from build123d import *

# Parameters (mm, degrees)
SKETCH_W        = 100
SKETCH_H        = 64
SKETCH_R        = 10.1
SKETCH_R_2      = 1.8
SKETCH_R_3      = 3.2
SKETCH_R_4      = 4
PAD_DEPTH       = 15
SKETCH001_R     = 11.2
SKETCH001_R_2   = 6
POCKET_DEPTH    = 6
SKETCH002_R     = 3.2
POCKET001_DEPTH = 3.2
SKETCH003_R     = 6
POCKET002_DEPTH = 6
SKETCH004_R     = 3.2
POCKET003_DEPTH = 15


with BuildPart() as part:
    # Sketch → Pad (new body)
    with BuildSketch(Plane.XY):
        with Locations((50, 32)):
            Rectangle(SKETCH_W, SKETCH_H)
        with Locations((50, 42.85)):
            Circle(SKETCH_R, mode=Mode.SUBTRACT)
        with Locations((65.5, 58.35)):
            Circle(SKETCH_R_2, mode=Mode.SUBTRACT)
        with Locations((65.5, 27.35)):
            Circle(SKETCH_R_2, mode=Mode.SUBTRACT)
        with Locations((34.5, 27.35)):
            Circle(SKETCH_R_2, mode=Mode.SUBTRACT)
        with Locations((34.5, 58.35)):
            Circle(SKETCH_R_2, mode=Mode.SUBTRACT)
        with Locations((20, 10)):
            Circle(SKETCH_R_3, mode=Mode.SUBTRACT)
        with Locations((80, 10)):
            Circle(SKETCH_R_3, mode=Mode.SUBTRACT)
        with Locations((82, 42.85)):
            Circle(SKETCH_R_4, mode=Mode.SUBTRACT)
        with Locations((18, 42.85)):
            Circle(SKETCH_R_4, mode=Mode.SUBTRACT)
    extrude(amount=PAD_DEPTH)

    # Sketch001 (on Face15 of Pad) → Pocket (cut)
    with BuildSketch(Plane.XY.offset(15)):
        with Locations((50, 42.85)):
            Circle(SKETCH001_R)
        with Locations((20, 10)):
            Circle(SKETCH001_R_2)
        with Locations((80, 10)):
            Circle(SKETCH001_R_2)
    extrude(amount=-POCKET_DEPTH, mode=Mode.SUBTRACT)

    # Sketch002 (on Face4 of Pocket) → Pocket001 (cut)
    with BuildSketch(Plane(origin=(0, 0, 0), x_dir=(1, 0, 0), z_dir=(0, 0, -1))):
        with Locations((34.5, -27.35)):
            Circle(SKETCH002_R)
        with Locations((65.5, -27.35)):
            Circle(SKETCH002_R)
        with Locations((34.5, -58.35)):
            Circle(SKETCH002_R)
        with Locations((65.5, -58.35)):
            Circle(SKETCH002_R)
    extrude(amount=-POCKET001_DEPTH, mode=Mode.SUBTRACT)

    # Sketch003 (on Face5 of Pocket001) → Pocket002 (cut)
    with BuildSketch(Plane.XY.offset(15)):
        with Locations((40, 10)):
            Circle(SKETCH003_R)
        with Locations((60, 10)):
            Circle(SKETCH003_R)
    extrude(amount=-POCKET002_DEPTH, mode=Mode.SUBTRACT)

    # Sketch004 (on Face4 of Pocket002) → Pocket003 (cut)
    with BuildSketch(Plane(origin=(0, 0, 0), x_dir=(1, 0, 0), z_dir=(0, 0, -1))):
        with Locations((40, -10)):
            Circle(SKETCH004_R)
        with Locations((60, -10)):
            Circle(SKETCH004_R)
    extrude(amount=-POCKET003_DEPTH, mode=Mode.SUBTRACT)


solid = part.part
Check sheet for the modelled part. Datum: model origin and axes. Units: mm. A direction names the side the tool comes from. Round coordinates to 2 decimals unless told otherwise and drop trailing zeros. Loops run counter-clockwise (first coordinate to the right, second up) from the corner with the lowest first, then second, coordinate; pieces in that order, holes last. Notation, with made-up numbers: (86.25, 40.5) - (140.25, 40.5) arc R22 cw to (140.25, 53.5) - close; hole circle Ø11 at (60, 32.25). An arc over 180 degrees is marked (long way). Answer as CSV lines item,"result". Start each with the question number.
Item 1: Section check A-A (x = 50). Record the boundary of the cut face in (y, z).
Item 2: Scan lines: line 1 (X direction, y = 27.35, z = 10.5); line 2 (X direction, y = 27.35, z = 2); line 3 (X direction, y = 10, z = 5). Record each from-to range of solid material in increasing order. Write a range as [from, to].
Item 3: Set-up check for faces 4 (the flat face through (63, 7, 9)), 5 (the cylindrical face through (62.961, 60.297, 1.578)), 6 (the cylindrical face through (56.8, 9.9, 4.4)): record each of +Z, -Z, +X, -X, +Y, -Y from which the full face is reachable in a straight line by a thin tool's end or side.
Item 4: Release check for a two-part mould opening along X. For faces 1 (the flat face through (49, 64, 7)), 2 (the cylindrical face through (22.769, 4.677, 12.042)), 3 (the flat face through (0, 32, 7)) record: +X half, -X half, draft (parallel to the pull), parting line (faces both ways), or undercut.
Item 5: Section check C-C (x = 82). Record the boundary of the cut face in (y, z).
Item 6: Section check B-B (y = 34). Record the boundary of the cut face in (x, z), and give its area (3 significant figures).
Item 7: Depth check by flat-ended pin: P1, Ø3, axis at x = 34.5, y = 58.35, coming from the +Z side; P2, Ø6, axis at x = 65.5, y = 58.35, coming from the -Z side. Enter the tip coordinate at first touch or a pass-through.
Item 8: Section check D-D (y = 10). Count the separate pieces of the cut face and the enclosed holes in it, and give its area (3 significant figures).
Report:
1,outline,"(0, 0) - (32.75, 0) - (32.75, 9) - (31.65, 9) - (31.65, 15) - (0, 15) - close; (52.95, 0) - (64, 0) - (64, 15) - (54.05, 15) - (54.05, 9) - (52.95, 9) - close"
2,line 1,"x = [0, 32.7], [36.3, 63.7], [67.3, 100]"
2,line 2,"x = [0, 31.3], [37.7, 62.3], [68.7, 100]"
2,line 3,"x = [0, 16.8], [23.2, 36.8], [43.2, 56.8], [63.2, 76.8], [83.2, 100]"
3,face 4,"+Z"
3,face 5,"-Z"
3,face 6,"+Z, -Z"
4,face 1,"draft"
4,face 2,"undercut"
4,face 3,"-X half"
5,outline,"(0, 0) - (7.5, 0) - (7.5, 9) - (4.34, 9) - (4.34, 15) - (0, 15) - close; (12.5, 0) - (38.85, 0) - (38.85, 15) - (15.66, 15) - (15.66, 9) - (12.5, 9) - close; (46.85, 0) - (64, 0) - (64, 15) - (46.85, 15) - close"
6,outline,"(0, 0) - (45.13, 0) - (45.13, 9) - (43.14, 9) - (43.14, 15) - (0, 15) - close; (54.87, 0) - (100, 0) - (100, 15) - (56.86, 15) - (56.86, 9) - (54.87, 9) - close"
6,area,"1,330 mm2"
7,P1,"passes through"
7,P2,"stops at z = 3.2"
8,separate pieces,"5"
8,enclosed holes,"0"
8,area,"982 mm2"
